For this review, take the finished solid that the model builds, in its own axes (mm). A direction names the side the tool comes from. Round coordinates to 2 decimals unless told otherwise and drop trailing zeros. Loops run counter-clockwise (first coordinate to the right, second up) from the corner with the lowest first, then second, coordinate; pieces in that order, holes last. Notation, with made-up numbers: M -23,64 L -8,64 A8 ccw -8,71 Z; hole C 10,36.5 d11. An arc over 180 degrees is marked long. One line per question, with ' | ' between items. Start each with the question number.
1) For probe 1 along Y at (x, z) = (13, 6.5); probe 2 along Z at (x, y) = (7.5, 48.5); probe 3 along Y at (x, z) = (11.75, 6.5), list the stretches that pass through material, from the lowest coordinate up. Write a range as from..to.
2) For pin 1 Ø12 at (x, y) = (3.5, 45.5) entering from +Z, flat-tipped, find the tip position at first contact; note if it passes through.
3) We need section B-B (y = 38.1). Give the boundary of the cut face in (x, z) (3 decimals).
4) Mouldability with a two-part tool opening along Y and no side actions: class faces 3 (the face through (12.437, 0.747, 0.156)), 4 (the face through (10.684, 65.046, 7.472)), 5 (the face through (13, 76.2, 3)) as pulls with the +Y half, pulls with the -Y half, needs draft (parallel to the pull), parting line crosses it, or undercut.
5) We need section D-D (z = 7.25). Give the boundary of the cut face in (x, y), and give its area (3 significant figures).
6) We need section A-A (x = 12.7). Give the boundary of the cut face in (y, z) (3 decimals).
7) For faces 1 (the face through (13, 64, 9.525)), 2 (the face through (12.15, 40.58, 7.47)), list the 3-axis set-ups (+Z, -Z, +X, -X, +Y, -Y) from which the entire face can be reached by the end or side of a thin tool; tool diameter is ignored.
8) We need section C-C (z = 1.75). Give the boundary of the cut face in (x, y).
Autodesk Fusion 360 part; units mm, degrees
sketch "Sketch1" plane through (0, 0, 0) normal (0, 0, 1) x (1, 0, 0)
  line L0 (0, 0) -> (25.4, 0)
  line L1 (25.4, 0) -> (25.4, 63.5)
  line L2 (25.4, 63.5) -> (0, 63.5) construction
  line L3 (0, 63.5) -> (0, 0)
  line L4 (25.4, 63.5) -> (25.4, 76.2)
  line L5 (25.4, 76.2) -> (0, 76.2)
  line L6 (0, 76.2) -> (0, 63.5)
  circle A0 centre (12.7, 63.5) radius 2.54
  circle A1 centre (12.7, 38.1) radius 2.54
  circle A2 centre (12.7, 12.7) radius 2.54
  circle A3 centre (12.7, 12.7) radius 12.7
  dimension "d8" = 25.4
  dimension "d9" = 63.5
  dimension "d11" = 12.7
  dimension "d12" = 5.08
  dimension "d15" = 25.4
  dimension "d16" = 0
extrude "Extrude1" add sketch "Sketch1" along normal blind 6.35 contours A3 | L1 L3 L4 L5 L6 A3 | A0 | A1 | A2
extrude "Extrude2" add sketch "Sketch1" along normal blind 3.175 from surface at 6.35 contours A0 | A1 | A2
chamfer "Chamfer1" distance 0.9 angle 45 9 edges at (10.3319, 11.7815, 9.525) (10.3319, 37.1815, 9.525) (10.3319, 62.5815, 9.525) (25.4, 76.2, 3.175) (0, 76.2, 3.175) (12.7, 76.2, 6.35) (0, 44.45, 6.35) (12.7, 0, 6.35) (25.4, 44.45, 6.35) 1 faces at (8.4667, 33.8667, 0)
equation "CUT_DISTANCE = 0.5 in"
equation "TUBE_WIDTH = 1 in"
equation "PIN_SPACING = 1 in"
equation "PIN_DIAMETER = 0.2 in"
equation "GUIDE_THICKNESS = 0.25 in"
equation "PIN_LENGTH = 0.125 in"
equation "PRINTER_LAYER_HEIGHT = 0.3 mm"
equation "d8 = TUBE_WIDTH"
equation "d9 = PIN_SPACING * ( PIN_COUNT - 0.5 )"
equation "d11 = CUT_DISTANCE"
equation "d12 = PIN_DIAMETER"
equation "d15 = PIN_SPACING"
equation "d17 = GUIDE_THICKNESS"
equation "d20 = PIN_LENGTH"
equation "d22 = PRINTER_LAYER_HEIGHT * 3"
Answers below:
1) probe 1: 10.18..15.22, 35.58..40.62, 60.98..66.02 | probe 2: 0..6.35 | probe 3: 10.34..15.06, 35.74..40.46, 61.14..65.86
2) pin 1: z = 6.35
3) outline: M 0,0.9 L 0.9,0 L 24.5,0 L 25.4,0.9 L 25.4,5.45 L 24.5,6.35 L 15.24,6.35 L 15.24,8.625 L 14.34,9.525 L 11.06,9.525 L 10.16,8.625 L 10.16,6.35 L 0.9,6.35 L 0,5.45 Z
4) face 3: pulls with the -Y half | face 4: undercut | face 5: pulls with the +Y half
5) outline: C 12.7,12.7 d5.08; C 12.7,38.1 d5.08; C 12.7,63.5 d5.08 | area: 60.8 mm^2
6) outline: M 0,0.9 L 0.9,0 L 75.3,0 L 76.2,0.9 L 76.2,5.45 L 75.3,6.35 L 66.04,6.35 L 66.04,8.625 L 65.14,9.525 L 61.86,9.525 L 60.96,8.625 L 60.96,6.35 L 40.64,6.35 L 40.64,8.625 L 39.74,9.525 L 36.46,9.525 L 35.56,8.625 L 35.56,6.35 L 15.24,6.35 L 15.24,8.625 L 14.34,9.525 L 11.06,9.525 L 10.16,8.625 L 10.16,6.35 L 0.9,6.35 L 0,5.45 Z
7) face 1: +Z, +X, -X, +Y, -Y | face 2: +Z
8) outline: M 0,12.7 A12.7 ccw 25.4,12.7 L 25.4,75.3 L 24.5,76.2 L 0.9,76.2 L 0,75.3 Z
